from build123d import *

# Parameters (mm, degrees)
SKETCH1_W            = 50
SKETCH1_H            = 150
BOSS_EXTRUDE1_DEPTH  = 1.524
SKETCH2_R            = 1.6
CUT_EXTRUDE1_DEPTH   = 1.524
LPATTERN1_COUNT      = 2
LPATTERN1_PITCH      = 44
LPATTERN1_COUNT_DIR2 = 2
LPATTERN1_PITCH_DIR2 = 134
FILLET1_R            = 4.191
SKETCH3_R            = 1.6
CUT_EXTRUDE2_DEPTH   = 1.524


with BuildPart() as part:
    # Sketch1 → Boss-Extrude1 (new body)
    with BuildSketch(Plane(origin=(0, 0, 0), x_dir=(1, 0, 0), z_dir=(0, 1, 0))):
        with Locations((25, -75)):
            Rectangle(SKETCH1_W, SKETCH1_H)
    extrude(amount=BOSS_EXTRUDE1_DEPTH)

    # Sketch2 → Cut-Extrude1 (cut)
    with BuildSketch(Plane(origin=(0, 1.524, 0), x_dir=(1, 0, 0), z_dir=(0, 1, 0))):
        with Locations((47, -8)):
            Circle(SKETCH2_R)
    cut_extrude1 = extrude(amount=-CUT_EXTRUDE1_DEPTH, mode=Mode.SUBTRACT)

    # LPattern1: Cut-Extrude1 2 × 2
    with Locations(*[(-i * LPATTERN1_PITCH, 0, j * LPATTERN1_PITCH_DIR2) for i in range(LPATTERN1_COUNT) for j in range(LPATTERN1_COUNT_DIR2) if (i, j) != (0, 0)]):
        add(cut_extrude1, mode=Mode.SUBTRACT)

    # Fillet1
    fillet1_edges = [part.edges().sort_by_distance(p)[0] for p in [
        (0, 0.762, 0),
        (50, 0.762, 0),
        (50, 0.762, 150),
        (0, 0.762, 150),
    ]]
    fillet(fillet1_edges, radius=FILLET1_R)

    # Sketch3 → Cut-Extrude2 (cut)
    with BuildSketch(Plane(origin=(0, 1.524, 0), x_dir=(1, 0, 0), z_dir=(0, 1, 0))):
        with Locations((25, -75)):
            Circle(SKETCH3_R)
    extrude(amount=-CUT_EXTRUDE2_DEPTH, mode=Mode.SUBTRACT)


solid = part.part
Can you work these out from the model? Positions are in its coordinate system, mm. Coordinates: 2 decimals unless noted, no trailing zeros. Order: outer loops, then holes, each group sorted by start corner. A loop starts at its lowest first (then second) coordinate and runs counter-clockwise, first axis right, second up. Notation, with made-up numbers: (78.5, 6.25) - (112.5, 6.25) arc R20 ccw to (112.5, 36.25) - close; hole circle Ø2 at (30, 24.5). An arc over 180 degrees is marked (long way). Answer as a JSON object with one key per item and string values. Group by question number.
Q1. Imagine slicing it at C-C (z = 75). Please give me the cut outline in (x, y), and give its area (3 significant figures).
Q2. Imagine slicing it at B-B (z = 142). Please give me the cut outline in (x, y).
Q3. We'd pull the mould along X, two halves only. Please class faces 1 (the face through (48.74, 0.773, 148.805)), 2 (the face through (3.74, 0.77, 143.42)), 3 (the face through (19, 1.524, 74)): +X half, -X half, draft (parallel to the pull), parting line (faces both ways), or undercut.
Q4. I need wall thicknesses on line 1 (X direction, y = 1.05, z = 8); line 2 (Z direction, x = 48, y = 0.7); line 3 (Z direction, x = 47, y = 0.7). Which ranges of each line are inside material? Lowest first, please. Write a range as from..to.
Q5. Imagine slicing it at A-A (x = 25). Please give me the cut outline in (y, z), and give its area (3 significant figures).
Determined:
{
 "1": {"outline": "(0, 0) - (23.4, 0) - (23.4, 1.52) - (0, 1.52) - close; (26.6, 0) - (50, 0) - (50, 1.52) - (26.6, 1.52) - close", "area": "71.3 mm2"},
 "2": {"outline": "(0, 0) - (1.4, 0) - (1.4, 1.52) - (0, 1.52) - close; (4.6, 0) - (45.4, 0) - (45.4, 1.52) - (4.6, 1.52) - close; (48.6, 0) - (50, 0) - (50, 1.52) - (48.6, 1.52) - close"},
 "3": {"face 1": "+X half", "face 2": "undercut", "face 3": "draft"},
 "4": {"line 1": "x = 0..1.4, 4.6..45.4, 48.6..50", "line 2": "z = 0.62..6.75, 9.25..140.75, 143.25..149.38", "line 3": "z = 0.17..6.4, 9.6..140.4, 143.6..149.83"},
 "5": {"outline": "(0, 0) - (1.52, 0) - (1.52, 73.4) - (0, 73.4) - close; (0, 76.6) - (1.52, 76.6) - (1.52, 150) - (0, 150) - close", "area": "224 mm2"}
}
